from build123d import *

# Parameters (mm, degrees)
SKETCH1_W                   = 19
SKETCH1_H                   = 18
BOSS_EXTRUDE1_DEPTH         = 32
TAP_DRILL_FOR_M3X0_5_TAP1_D = 2.5
FILLET1_R                   = 2


with BuildPart() as part:
    # Sketch1 → Boss-Extrude1 (new body)
    with BuildSketch(Plane(origin=(0, 0, 0), x_dir=(1, 0, 0), z_dir=(0, 1, 0))):
        with Locations((9.5, 9)):
            Rectangle(SKETCH1_W, SKETCH1_H)
        Polygon((4, 4), (15, 4), (15, 11.5), (9.5, 17), (4, 11.5), align=None, mode=Mode.SUBTRACT)
    extrude(amount=BOSS_EXTRUDE1_DEPTH)

    # Tap Drill for M3x0.5 Tap1 (through all)
    with Locations(Plane(origin=(19, 0, 0), x_dir=(0, 0, -1), z_dir=(1, 0, 0))):
        with Locations((8.419226219, 28.375), (8.419226219, 3.625)):
            Hole(TAP_DRILL_FOR_M3X0_5_TAP1_D / 2)

    # Fillet1
    fillet1_edges = [part.edges().sort_by_distance(p)[0] for p in [
        (0, 16, -18),
        (19, 16, -18),
        (19, 16, 0),
        (0, 16, 0),
    ]]
    fillet(fillet1_edges, radius=FILLET1_R)

    # Sketch5 → M5 Clearance Hole1 (revolve, cut)
    with BuildSketch(Plane(origin=(9.744397645, 16.5210513, 0), x_dir=(0, -1, 0), z_dir=(1, 0, 0))):
        Polygon((0, 0), (0, 4), (2.55, 4), (2.55, 0.571259203), (2.95, 0), align=None)
    revolve(axis=Axis((9.744397645, 16.5210513, 6.35), (0, 0, -1)), mode=Mode.SUBTRACT)


solid = part.part
Design review of the part built by this model. Coordinates are the model's own, in mm. A direction names the side the tool comes from. Round coordinates to 2 decimals unless told otherwise and drop trailing zeros. Write each loop counter-clockwise with the first axis right and the second up, starting at its lowest first coordinate (ties: lowest second). Pieces come first, ordered by that corner, then holes. Notation, with made-up numbers: (49, 42) - (83, 42) arc R25 cw to (83, 81) - close; hole circle Ø1 at (23, 50.5). An arc over 180 degrees is marked (long way). Use a Markdown table: item, result. Add a question column.
1. We need section A-A (z = -14.75). State the section outline as (x, y) points.
2. For faces 1 (the face through (18.4, 16.22, -17.43)), 2 (the face through (7.216, 16.853, -2.262)), 3 (the face through (6.8, 15.8, -14.3)), list the 3-axis set-ups (+Z, -Z, +X, -X, +Y, -Y) from which the entire face can be reached by the end or side of a thin tool; tool diameter is ignored.
3. Mouldability with a two-part tool opening along Y and no side actions: class faces 4 (the face through (9, 16, -18)), 5 (the face through (5, 0, -13)), 6 (the face through (1.97, 2.86, -9.41)) as +Y half, -Y half, draft (parallel to the pull), parting line (faces both ways), or undercut.
4. Wall thickness on probe 1 along X at (y, z) = (8, -10); probe 2 along Y at (x, z) = (1.5, -7.75); probe 3 along Z at (x, y) = (8.5, 20.5): over which ranges is each line inside the solid? List them lowest first.
5. We need section D-D (x = 16). State the section outline as (y, z) points (3 decimals).
6. We need section B-B (y = 7). State the section outline as (x, z) points.
7. Clearance check with a flat-ended pin moving along its axis: pin 1 (2 mm diameter, centred on y = 3.62, z = -8.42, fed in from -X). State where the tip first meets the part, or that it passes through.
8. We need section C-C (x = 4.5). State the section outline as (y, z) points.
Output:
| question | item | result |
|---|---|---|
| 1 | outline | (0, 0) - (7.25, 0) - (7.25, 32) - (0, 32) - close; (11.75, 0) - (19, 0) - (19, 32) - (11.75, 32) - close |
| 2 | face 1 | -Z, +X, +Y, -Y |
| 2 | face 2 | +Z |
| 2 | face 3 | +Y, -Y |
| 3 | face 4 | draft |
| 3 | face 5 | -Y half |
| 3 | face 6 | undercut |
| 4 | probe 1 | x = 0 to 4, 15 to 19 |
| 4 | probe 2 | y = 0 to 2.57, 4.68 to 27.32, 29.43 to 32 |
| 4 | probe 3 | z = -18 to -16, -4 to 0 |
| 5 | outline | (0, -18) - (32, -18) - (32, 0) - (0, 0) - close; hole circle Ø2.5 at (3.625, -8.419); hole circle Ø2.5 at (28.375, -8.419) |
| 6 | outline | (0, -16) arc R2 ccw to (2, -18) - (17, -18) arc R2 ccw to (19, -16) - (19, -2) arc R2 ccw to (17, 0) - (2, 0) arc R2 ccw to (0, -2) - close; hole (4, -11.5) - (9.5, -17) - (15, -11.5) - (15, -4) - (4, -4) - close |
| 7 | pin 1 | passes through |
| 8 | outline | (0, -18) - (32, -18) - (32, -12) - (0, -12) - close; (0, -4) - (32, -4) - (32, 0) - (0, 0) - close |
